Here's the drawing with two shaded views (mm, measured from the low corner). I have some questions. Coordinates: 2 decimals unless noted, no trailing zeros. Write each loop counter-clockwise with the first axis right and the second up, starting at its lowest first coordinate (ties: lowest second). Pieces come first, ordered by that corner, then holes. Notation, with made-up numbers: (-29.5, 66.25) - (-5.5, 66.25) arc R23 cw to (-5.5, 99.25) - close; hole circle Ø5 at (14, -8). An arc over 180 degrees is marked (long way). Answer in a Markdown table with one row per item. Add a question column.
Item 1: Imagine slicing it at C-C (y = 1.1). Please give me the cut outline in (x, z).
Item 2: Imagine slicing it at A-A (z = 32.5). Please give me the cut outline in (x, y), plus the area to 3 significant figures.
Item 3: Imagine slicing it at B-B (x = 63.45). Please give me the cut outline in (y, z).
Item 4: I'm going to push a flat-ended pin straight in: pin 1 (8.5 mm diameter, centred on x = 11.55, z = 57.5, fed in from +Y). Where does the tip first touch, or does it pass through?
Item 5: If I drill on probe 1 along Z at (x, y) = (63.45, 0.7); probe 2 along X at (y, z) = (0.95, 7.5); probe 3 along Z at (x, y) = (67.5, 0.9), over which ranges is the centre line in solid material (lowest first)? Write a range as from..to.
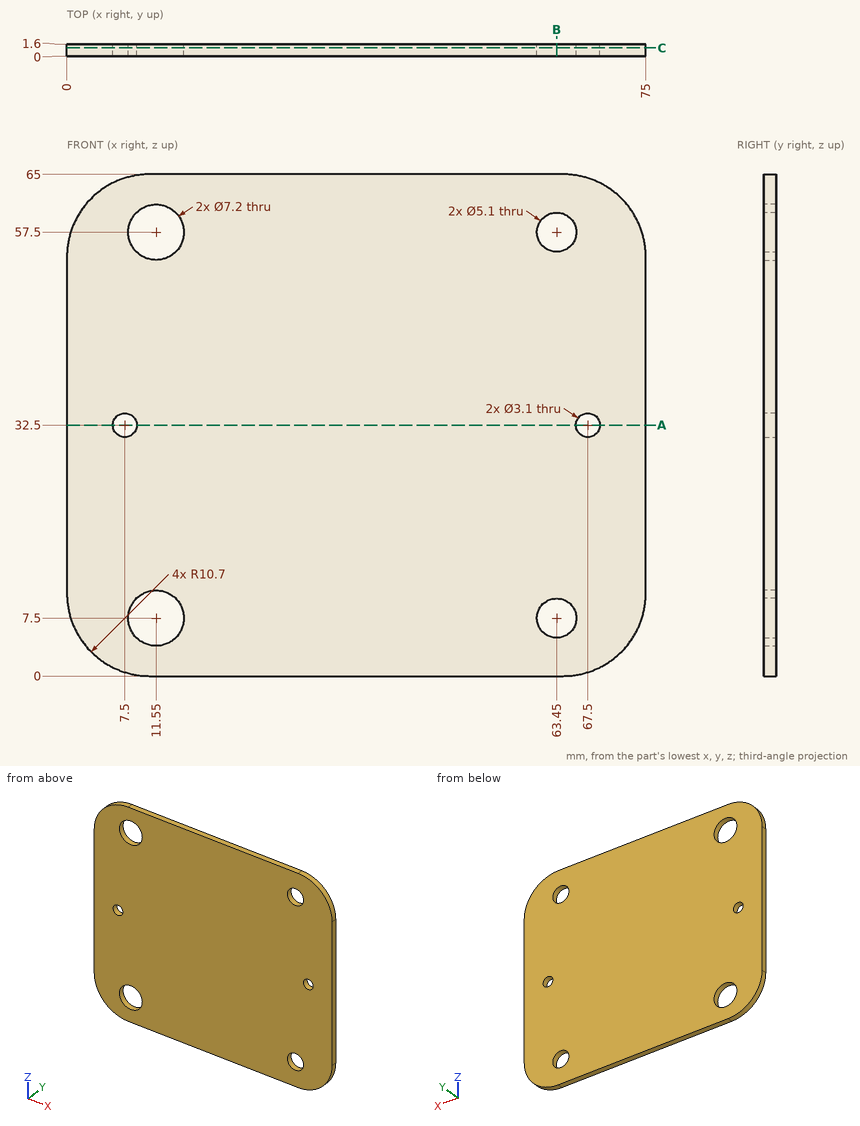
Here are the results:
| question | item | result |
|---|---|---|
| 1 | outline | (0, 10.7) arc R10.7 ccw to (10.7, 0) - (64.3, 0) arc R10.7 ccw to (75, 10.7) - (75, 54.3) arc R10.7 ccw to (64.3, 65) - (10.7, 65) arc R10.7 ccw to (0, 54.3) - close; hole circle Ø3.1 at (7.5, 32.5); hole circle Ø7.2 at (11.55, 7.5); hole circle Ø7.2 at (11.55, 57.5); hole circle Ø5.1 at (63.45, 7.5); hole circle Ø5.1 at (63.45, 57.5); hole circle Ø3.1 at (67.5, 32.5) |
| 2 | outline | (0, 0) - (5.95, 0) - (5.95, 1.6) - (0, 1.6) - close; (9.05, 0) - (65.95, 0) - (65.95, 1.6) - (9.05, 1.6) - close; (69.05, 0) - (75, 0) - (75, 1.6) - (69.05, 1.6) - close |
| 2 | area | 110 mm2 |
| 3 | outline | (0, 0) - (1.6, 0) - (1.6, 4.95) - (0, 4.95) - close; (0, 10.05) - (1.6, 10.05) - (1.6, 54.95) - (0, 54.95) - close; (0, 60.05) - (1.6, 60.05) - (1.6, 65) - (0, 65) - close |
| 4 | pin 1 | stops at y = 1.6 |
| 5 | probe 1 | z = 0..4.95, 10.05..54.95, 60.05..65 |
| 5 | probe 2 | x = 0.49..7.95, 15.15..60.9, 66..74.51 |
| 5 | probe 3 | z = 0.49..30.95, 34.05..64.51 |
